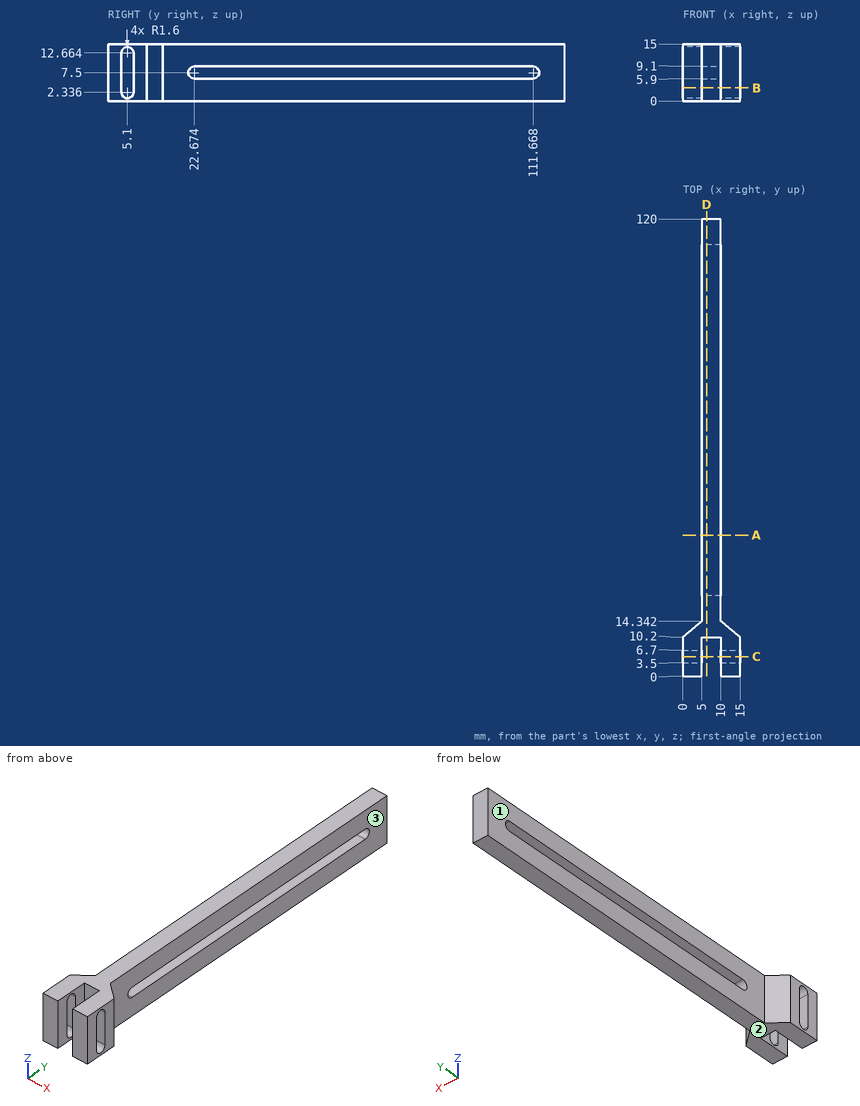
Geometry check sheet. Reference: drawing and pictorial views, mm from the part's lowest x, y, z. A direction names the side the tool comes from. Coordinates: 2 decimals unless noted, no trailing zeros. Order: outer loops, then holes, each group sorted by start corner. A loop starts at its lowest first (then second) coordinate and runs counter-clockwise, first axis right, second up.
Item 1: Depth check by flat-ended pin: pin 1 (8 mm diameter, centred on y = 100, z = 1.5, fed in from +X); pin 2 (1.5 mm diameter, centred on x = 2, z = 8.5, fed in from +Y); pin 3 (4 mm diameter, centred on y = 32.5, z = 6, fed in from -X). Enter the tip coordinate at first touch or a pass-through.
Item 2: Section check B-B (z = 3.5). Enter the section's corners in (x, y).
Item 3: Scan lines: line 1 along Z through (x, y) = (5.75, 23.5); line 2 along X through (y, z) = (52, 2.25); line 3 along Y through (x, z) = (11, 9) (1 decimal). Record each from-to range of solid material in increasing order.
Item 4: Tool access check on the marked faces 1, 2 and 3. Record the directions out of +Z, -Z, +X, -X, +Y, -Y that give a thin tool (end or side, any length) a straight path to the whole face; none if there is none.
Item 5: Section check C-C (y = 5.1). Enter the section's corners in (x, z).
Item 6: Section check A-A (y = 37). Enter the section's corners in (x, z), plus the area to 3 significant figures.
Item 7: Section check D-D (x = 6.25). Enter the section's corners in (y, z).
Check sheet entries:
1. pin 1: stops at x = 10
1. pin 2: stops at y = 12.48
1. pin 3: stops at x = 5
2. outline: (0, 0) - (5, 0) - (5, 3.5) - (0, 3.5) - close; (0, 6.7) - (5, 6.7) - (5, 10.2) - (10, 10.2) - (10, 6.7) - (15, 6.7) - (15, 10.2) - (10, 14.34) - (10, 120) - (5, 120) - (5, 14.34) - (0, 10.2) - close; (10, 0) - (15, 0) - (15, 3.5) - (10, 3.5) - close
3. line 1: z = 0 to 5.9, 9.1 to 15
3. line 2: x = 5 to 10
3. line 3: y = 0 to 3.5, 6.7 to 13.5
4. face 1: +Z, -Z, -X, +Y
4. face 2: -Z, +X, -X, +Y, -Y
4. face 3: +Z, -Z, +X, +Y
5. outline: (0, 0) - (5, 0) - (5, 0.74) - (0, 0.74) - close; (0, 14.26) - (5, 14.26) - (5, 15) - (0, 15) - close; (10, 0) - (15, 0) - (15, 0.74) - (10, 0.74) - close; (10, 14.26) - (15, 14.26) - (15, 15) - (10, 15) - close
6. outline: (5, 0) - (10, 0) - (10, 5.9) - (5, 5.9) - close; (5, 9.1) - (10, 9.1) - (10, 15) - (5, 15) - close
6. area: 59.0 mm2
7. outline: (10.2, 0) - (120, 0) - (120, 15) - (10.2, 15) - close; hole (22.67, 5.9) - (111.67, 5.9) arc R1.6 ccw to (111.67, 9.1) - (22.67, 9.1) arc R1.6 ccw to start
